from build123d import *

# Parameters (mm, degrees)
F0_W     = 23
F0_H     = 54.175
F0_W_2   = 4
F0_H_2   = 3.175
F0_W_3   = 17
F0_H_3   = 18
F0_W_4   = 10
F0_H_4   = 10
F0_R     = 1.2
F1_DEPTH = 3.175


# Not quite as in the source:
# - a length typed as a fraction of an inch, garbled in the dataset ("3 / 203.2 mm" for 3/8 in), is restored
# - a feature names something its author has since deleted; it is built from what else it names


with BuildPart() as f1:
    # F0 (on Top) → F1 (new body)
    with BuildSketch(Plane.XY):
        with Locations((11.4247928681, 25.3005515426)):
            Rectangle(F0_W, F0_H)
        with Locations((4.9247928681, 3.8005515426)):
            Rectangle(F0_W_2, F0_H_2, mode=Mode.SUBTRACT)
        with BuildLine():
            ThreePointArc((11.4247928681, 5.3005515426), (12.4854530398, 4.8612117144), (12.9247928681, 3.8005515426))
            ThreePointArc((12.9247928681, 3.8005515426), (10.3641326963, 2.7398913709), (11.4247928681, 5.3005515426))
        make_face(mode=Mode.SUBTRACT)
        with Locations((17.9247928681, 3.8005515426)):
            Rectangle(F0_W_2, F0_H_2, mode=Mode.SUBTRACT)
        with Locations((11.4247928681, 17.3880515426)):
            Rectangle(F0_W_3, F0_H_3, mode=Mode.SUBTRACT)
        Polygon((6.4247928681, 29.3880515426), (6.4247928681, 39.3880515426), (6.4247928681, 49.3880515426), (16.4247928681, 49.3880515426), (16.4247928681, 39.3880515426), (16.4247928681, 29.3880515426), align=None, mode=Mode.SUBTRACT)
        with Locations((11.4247928681, 34.3880515426)):
            Rectangle(F0_W_4, F0_H_4)
        with Locations((11.4247928681, 34.3880515426)):
            Circle(F0_R, mode=Mode.SUBTRACT)
    extrude(amount=F1_DEPTH)


solid = f1.part
Here's how the part is built. I have some questions about the finished solid (model axes, mm). A direction names the side the tool comes from. Round coordinates to 2 decimals unless told otherwise and drop trailing zeros. Loops run counter-clockwise (first coordinate to the right, second up) from the corner with the lowest first, then second, coordinate; pieces in that order, holes last. Notation, with made-up numbers: M -15,29.25 L 21,29.25 A18 ccw 21,62.25 Z; hole C 2.5,-32.75 d6. An arc over 180 degrees is marked long. Write each question's results on one line, items separated by ' | '. Start each with the question number.
(1) I want a section at D-D (x = 19). Please give me the cut outline in (y, z) (3 decimals), then the cut area to 3 significant figures.
(2) I want a section at B-B (x = 15). Please give me the cut outline in (y, z) (3 decimals).
(3) Will this pin go through, and if not, where does the flat tip stop? P1, Ø4, axis at x = 3, y = 21.5, coming from the +Z side (3 decimals).
(4) On a 3-axis mill with a long thin cutter (end or side, diameter ignored), from which of +Z, -Z, +X, -X, +Y, -Y can I reach the whole of each face in a straight line? I mean faces 4 (the flat face through (5, 5.388, 2)), 5 (the flat face through (-0.075, 25, 2)). Say none if no direction works.
(5) Thinking about a two-plate mould opening in Y: for faces 1 (the flat face through (11, -1.787, 2)), 2 (the flat face through (19.925, 4, 2)), 3 (the flat face through (22.925, 25, 2)), which applies, pulls with the +Y half, pulls with the -Y half, needs draft (parallel to the pull), parting line crosses it, or undercut?
(6) I want a section at C-C (z = 1.45). Please give me the cut outline in (x, y).
(7) I want a section at A-A (y = 15). Please give me the cut outline in (x, z) (3 decimals).
(8) If I drill on probe 1 along Y at (x, z) = (9.75, 2.9); probe 2 along Y at (x, z) = (5.5, 2.7); probe 3 along X at (y, z) = (23, 0.7), over which ranges is the centre line in solid material (lowest first)? Write a range as from..to.
Solved:
1) outline: M -1.787,0 L 2.213,0 L 2.213,3.175 L -1.787,3.175 Z; M 5.388,0 L 8.388,0 L 8.388,3.175 L 5.388,3.175 Z; M 26.388,0 L 52.388,0 L 52.388,3.175 L 26.388,3.175 Z | area: 105 mm²
2) outline: M -1.787,0 L 8.388,0 L 8.388,3.175 L -1.787,3.175 Z; M 26.388,0 L 39.388,0 L 39.388,3.175 L 26.388,3.175 Z; M 49.388,0 L 52.388,0 L 52.388,3.175 L 49.388,3.175 Z
3) P1: stops at z = 3.175
4) face 4: +Z, -Z | face 5: +Z, -Z, -X, +Y, -Y
5) face 1: pulls with the -Y half | face 2: undercut | face 3: needs draft
6) outline: M -0.08,-1.79 L 22.92,-1.79 L 22.92,52.39 L -0.08,52.39 Z; hole M 2.92,2.21 L 6.92,2.21 L 6.92,5.39 L 2.92,5.39 Z; hole M 2.92,8.39 L 19.92,8.39 L 19.92,26.39 L 2.92,26.39 Z; hole M 6.42,39.39 L 16.42,39.39 L 16.42,49.39 L 6.42,49.39 Z; hole C 11.42,3.8 d3; hole C 11.42,34.39 d2.4; hole M 15.92,2.21 L 19.92,2.21 L 19.92,5.39 L 15.92,5.39 Z
7) outline: M -0.075,0 L 2.925,0 L 2.925,3.175 L -0.075,3.175 Z; M 19.925,0 L 22.925,0 L 22.925,3.175 L 19.925,3.175 Z
8) probe 1: y = -1.79..8.39, 26.39..39.39, 49.39..52.39 | probe 2: y = -1.79..2.21, 5.39..8.39, 26.39..52.39 | probe 3: x = -0.08..2.92, 19.92..22.92
